Autodesk Inventor part; units mm, degrees
ref_plane "YZ Plane" through (0, 0, 0) normal (1, 0, 0) x (0, 1, 0)
ref_plane "XZ Plane" through (0, 0, 0) normal (0, 1, 0) x (-1, 0, 0)
ref_plane "XY Plane" through (0, 0, 0) normal (0, 0, 1) x (1, 0, 0)
sketch "Sketch1" plane through (0, 0, 0) normal (0, 1, 0) x (-1, 0, 0)
  circle A0 centre (-15.24, 2.54) radius 2
  circle A1 centre (-66.04, 17.78) radius 2
  circle A2 centre (-66.04, 45.72) radius 2
  circle A3 centre (-15.24, 50.8) radius 2
  line L0 (0, 0) -> (-68.58, 0) construction
  line L1 (-68.58, 0) -> (-68.58, 53.34) construction
  line L2 (-68.58, 53.34) -> (0, 53.34) construction
  line L3 (0, 53.34) -> (0, 0) construction
  line L4 (-68.58, -1.27) -> (0, -1.27)
  line L5 (1.27, 0) -> (1.27, 53.34)
  line L6 (0, 54.61) -> (-68.58, 54.61)
  line L7 (-69.85, 53.34) -> (-69.85, 0)
  arc A4 (0, -1.27) -> (1.27, 0) centre (0, 0) ccw
  arc A5 (-69.85, 0) -> (-68.58, -1.27) centre (-68.58, 0) ccw
  arc A6 (-68.58, 54.61) -> (-69.85, 53.34) centre (-68.58, 53.34) ccw
  arc A7 (1.27, 53.34) -> (0, 54.61) centre (0, 53.34) ccw
  arc A8 (-11.335, 2.54) -> (-19.145, 2.54) centre (-15.24, 2.54) ccw
  arc A9 (-19.145, 50.8) -> (-11.335, 50.8) centre (-15.24, 50.8) ccw
  arc A10 (-66.04, 41.815) -> (-66.04, 49.625) centre (-66.04, 45.72) ccw
  arc A11 (-66.04, 13.875) -> (-66.04, 21.685) centre (-66.04, 17.78) ccw
  line L8 (-11.335, 2.54) -> (-19.145, 2.54) construction
  line L9 (-19.145, 2.54) -> (-19.145, -1.27)
  line L10 (-19.145, -1.27) -> (-11.335, -1.27)
  line L11 (-11.335, -1.27) -> (-11.335, 2.54)
  line L12 (-66.04, 13.875) -> (-69.85, 13.875)
  line L13 (-69.85, 13.875) -> (-69.85, 21.685)
  line L14 (-69.85, 21.685) -> (-66.04, 21.685)
  line L15 (-66.04, 21.685) -> (-66.04, 13.875) construction
  line L16 (-66.04, 41.815) -> (-69.85, 41.815)
  line L17 (-69.85, 41.815) -> (-69.85, 49.625)
  line L18 (-69.85, 49.625) -> (-66.04, 49.625)
  line L19 (-66.04, 49.625) -> (-66.04, 41.815) construction
  line L20 (-19.145, 50.8) -> (-11.335, 50.8) construction
  line L21 (-11.335, 50.8) -> (-11.335, 54.61)
  line L22 (-11.335, 54.61) -> (-19.145, 54.61)
  line L23 (-19.145, 54.61) -> (-19.145, 50.8)
  dimension "d0" = 4
  dimension "d4" = 15.24
  dimension "d5" = 2.54
  dimension "d6" = 17.78
  dimension "d7" = 66.04
  dimension "d8" = 45.72
  dimension "d9" = 50.8
  dimension "d10" = 2.54
  dimension "d11" = 2.54
  dimension "d12" = 1.27
  dimension "d13" = 1.27
  dimension "d14" = 1.905
extrude "Extrusion1" add sketch "Sketch1" along normal blind 6 contours L9 A8 L11 L4 | L7 L14 A11 L12 | L7 L18 A10 L16 | L21 A9 L23 L6
extrude "Extrusion2" add sketch "Sketch1" against normal blind 2 contours A0 | A1 | A2 | A3 | A5 L7 L12 A11 L14 L16 A10 L18 A6 L6 L23 A9 L21 A7 L5 A4 L4 L11 A8 L9 | L9 A8 L11 L4 | L7 L14 A11 L12 | L7 L18 A10 L16 | L21 A9 L23 L6
sketch "Sketch2" plane through (0, -2, 0) normal (0, -1, 0) x (1, 0, 0)
  line L0 (68.58, 54.61) -> (0, 54.61)
  arc A0 (0, 54.61) -> (-1.27, 53.34) centre (0, 53.34) ccw
  line L1 (-1.27, 53.34) -> (-1.27, 0)
  arc A1 (-1.27, 0) -> (0, -1.27) centre (0, 0) ccw
  line L2 (0, -1.27) -> (68.58, -1.27)
  arc A2 (68.58, -1.27) -> (69.85, 0) centre (68.58, 0) ccw
  line L3 (69.85, 0) -> (69.85, 53.34)
  arc A3 (69.85, 53.34) -> (68.58, 54.61) centre (68.58, 53.34) ccw
  line L4 (68.58, -2.8575) -> (0, -2.8575)
  arc A4 (-2.8575, 0) -> (0, -2.8575) centre (0, 0) ccw
  line L5 (-2.8575, 0) -> (-2.8575, 53.34)
  arc A5 (0, 56.1975) -> (-2.8575, 53.34) centre (0, 53.34) ccw
  line L6 (0, 56.1975) -> (68.58, 56.1975)
  arc A6 (71.4375, 53.34) -> (68.58, 56.1975) centre (68.58, 53.34) ccw
  line L7 (71.4375, 53.34) -> (71.4375, 0)
  arc A7 (68.58, -2.8575) -> (71.4375, 0) centre (68.58, 0) ccw
  point P0 (0, 0)
  dimension "d19" = 1.5875
extrude "Extrusion3" add sketch "Sketch2" against normal blind 27.05
sketch "Sketch4" plane through (-2.8575, -2, 0) normal (-1, 0, 0) x (0, 0, 1)
  line L0 (2.54, 8) -> (-1.27, 8)
  line L1 (-1.27, 8) -> (2.54, 8)
  line L2 (2.54, 8) -> (2.54, 8)
  line L3 (0.54, 8) -> (4.54, 8)
  line L4 (0, 2) -> (53.34, 2)
  line L5 (50.8, 8) -> (54.61, 8)
  line L6 (54.61, 8) -> (50.8, 8)
  line L7 (50.8, 8) -> (50.8, 8)
  line L8 (48.8, 8) -> (52.8, 8)
  line L9 (0, 27.05) -> (53.34, 27.05)
  line L10 (50.8, 8) -> (54.61, 8)
  line L11 (50.8, 8) -> (46.895, 8)
  line L12 (50.8, 8) -> (50.8, 20.7)
  line L13 (50.8, 20.7) -> (39.6875, 20.7) construction
  line L14 (43.72, 8) -> (47.72, 8)
  line L15 (39.6875, 20.7) -> (39.6875, 8)
  line L16 (39.6875, 8) -> (50.8, 8)
  ellipse E0 centre (45.2438, 20.7) end of major axis (50.8, 20.7) minor radius 2.54 (50.8, 20.7) -> (39.6875, 20.7) ccw
  ellipse E1 centre (45.2438, 20.7) end of major axis (50.8, 20.7) minor radius 2.54 (39.6875, 20.7) -> (50.8, 20.7) ccw construction
  line L17 (10.3188, 8) -> (10.3188, 20.7)
  line L18 (10.3188, 8) -> (23.0188, 8)
  line L19 (15.78, 8) -> (19.78, 8)
  line L20 (23.0188, 8) -> (23.0188, 20.7)
  ellipse E2 centre (16.6688, 20.7) end of major axis (23.0188, 20.7) minor radius 2.54 (23.0188, 20.7) -> (10.3188, 20.7) ccw
  point P0 (2.54, 2)
  point P1 (2.54, 2)
  point P2 (2.54, 2)
  point P3 (50.8, 2)
  point P4 (2.54, 2)
  point P5 (16.6688, 8)
  dimension "d26" = 2.54
  dimension "d29" = 2.54
  dimension "d24" = 12.7
  dimension "d25" = 11.1125
  dimension "d27" = 10.3187
  dimension "d28" = 12.7
extrude "Extrusion5" cut sketch "Sketch4" against normal up to surface (1.5875 mm away)
sketch "Sketch5" plane through (0, -2, 0) normal (0, -1, 0) x (1, 0, 0)
  line L0 (68.58, 56.1975) -> (0, 56.1975)
  arc A0 (0, 56.1975) -> (-2.8575, 53.34) centre (0, 53.34) ccw
  line L1 (-2.8575, 53.34) -> (-2.8575, 0)
  arc A1 (-2.8575, 0) -> (0, -2.8575) centre (0, 0) ccw
  line L2 (0, -2.8575) -> (68.58, -2.8575)
  arc A2 (68.58, -2.8575) -> (71.4375, 0) centre (68.58, 0) ccw
  line L3 (71.4375, 0) -> (71.4375, 53.34)
  arc A3 (71.4375, 53.34) -> (68.58, 56.1975) centre (68.58, 53.34) ccw
  line L4 (0, 56.1975) -> (68.58, 56.1975)
  line L5 (0, 56.1975) -> (12.7, 56.1975)
  line L6 (12.7, 56.1975) -> (12.7, 59.3725)
  line L7 (0, 62.5475) -> (0, 62.5475)
  line L8 (0, 62.5475) -> (0, 56.1975)
  line L9 (68.58, 56.1975) -> (55.88, 56.1975)
  line L10 (55.88, 56.1975) -> (55.88, 62.5475)
  line L11 (55.88, 62.5475) -> (55.88, 62.5475)
  line L12 (68.58, 59.3725) -> (68.58, 56.1975)
  line L13 (0, -2.8575) -> (12.7, -2.8575)
  line L14 (12.7, -2.8575) -> (12.7, -6.0325)
  line L15 (0, -9.2075) -> (0, -9.2075)
  line L16 (0, -9.2075) -> (0, -2.8575)
  line L17 (68.58, -2.8575) -> (0, -2.8575)
  line L18 (68.58, -2.8575) -> (55.88, -2.8575)
  line L19 (55.88, -2.8575) -> (55.88, -9.2075)
  line L20 (55.88, -9.2075) -> (55.88, -9.2075)
  line L21 (68.58, -6.0325) -> (68.58, -2.8575)
  line L22 (12.7, 59.3725) -> (0, 62.5475)
  line L23 (55.88, 62.5475) -> (68.58, 59.3725)
  line L24 (12.7, -6.0325) -> (0, -9.2075)
  line L25 (55.88, -9.2075) -> (68.58, -6.0325)
  point P0 (0, 0)
  point P1 (12.7, 62.5475)
  point P2 (68.58, 62.5475)
  point P3 (12.7, -9.2075)
  point P4 (68.58, -9.2075)
  dimension "d32" = 12.7
  dimension "d33" = 6.35
  dimension "d34" = 12.7
  dimension "d35" = 6.35
  dimension "d36" = 12.7
  dimension "d37" = 6.35
  dimension "d38" = 12.7
  dimension "d39" = 6.35
  dimension "d40" = 3.175
  dimension "d41" = 12.7
  dimension "d42" = 12.7
  dimension "d43" = 3.175
  dimension "d44" = 3.175
  dimension "d45" = 12.7
  dimension "d46" = 12.7
  dimension "d47" = 3.175
extrude "Extrusion6" add sketch "Sketch5" against normal blind 3.175 contours L0 L10 L23 L12 | L0 L8 L22 L6 | L21 L25 L19 L2 | L14 L24 L16 L2
properties part number "ArduinoHolder-v1"
Input: part model. Units: mm. Frame: model coordinates. A direction names the side the tool comes from. Coordinates: 2 decimals unless noted, no trailing zeros. Write each loop counter-clockwise with the first axis right and the second up, starting at its lowest first coordinate (ties: lowest second). Pieces come first, ordered by that corner, then holes.
1) Material intervals for line 1 along Z through (x, y) = (66.04, 1.95) (1 decimal); line 2 along Z through (x, y) = (15.24, 2.05) (1 decimal); line 3 along Z through (x, y) = (4.5, 16.5), sorted ascending.
2) Section C-C on z = 36. Output: boundary loops of the cut face in (x, y).
3) Mould query, pull axis Z, two halves, no side actions, for faces 4 (the flat face through (68, 3, 13.875)), 5 (the flat face through (62.141, -0.435, -7.642)), 6 (the flat face through (55.88, 0, -6)). Classes: pulls with the +Z half, pulls with the -Z half, needs draft (parallel to the pull), parting line crosses it, or undercut.
4) Set-up query: faces 1 (the flat face through (11.335, 3, 53)), 2 (the flat face through (62, 1.175, -5)), 3 (the flat face through (68, 6, 16)). Return all of +Z, -Z, +X, -X, +Y, -Y with unobstructed straight access to the full face (end or side cutting, diameter ignored); none if empty.
5) Pin query (flat end, axial travel): pin 1 Ø1.3 at (x, y) = (-2, 13) entering from +Z; pin 2 Ø4 at (x, y) = (68.5, 4) entering from +Z; pin 3 Ø3.5 at (y, z) = (0, -6) entering from -X. Return the tip coordinate at first contact, or that it passes through.
6) Section A-A on x = 55. Output: boundary loops of the cut face in (y, z).
Check result:
1. line 1: z = -2.9 to -1.3, 13.9 to 15.8, 19.8 to 21.7, 41.8 to 43.7, 47.7 to 49.6, 54.6 to 56.2
1. line 2: z = -2.9 to 0.5, 4.5 to 6.4, 46.9 to 48.8, 52.8 to 56.2
1. line 3: z = -2.86 to -1.27, 54.61 to 56.2
2. outline: (-2.86, -2) - (71.44, -2) - (71.44, 25.05) - (69.85, 25.05) - (69.85, 0) - (-1.27, 0) - (-1.27, 25.05) - (-2.86, 25.05) - close
3. face 4: undercut
3. face 5: pulls with the -Z half
3. face 6: needs draft
4. face 1: +Y
4. face 2: -Z, +X, -X, +Y
4. face 3: -X, +Y
5. pin 1: stops at z = 55.86
5. pin 2: stops at z = 56.2
5. pin 3: stops at x = 0
6. outline: (-2, -2.86) - (25.05, -2.86) - (25.05, -1.27) - (0, -1.27) - (0, 54.61) - (25.05, 54.61) - (25.05, 56.2) - (-2, 56.2) - close
